```python
from build123d import *

# Parameters (mm, degrees)
SKETCH_2_W        = 3
SKETCH_2_H        = 6
EXTRUDE_660_DEPTH = 5


with BuildPart() as part:
    # Sketch 202 → Revolve 495 (revolve)
    with BuildSketch(Plane.XY, mode=Mode.PRIVATE) as revolve_495_sk:
        with BuildLine():
            Line((15, 0), (13, 0))
            Line((13, 0), (6, 10))
            Line((6, 10), (0, 10))
            Line((0, 10), (0, 286.3))
            Line((0, 286.3), (10, 286.3))
            ThreePointArc((10, 286.3), (14.127651137, 284.674598502), (18, 282.510262985))
            Line((18, 282.510262985), (18, 285.510262985))
            Line((18, 285.510262985), (20, 285.510262985))
            Line((20, 285.510262985), (20, 281.10043911))
            ThreePointArc((20, 281.10043911), (29.571946165, 269.497448129), (33, 254.851629613))
            Line((33, 254.851629613), (33, 39.851629613))
            ThreePointArc((33, 39.851629613), (27.867639585, 22.176939688), (14.066990064, 10))
            Line((14.066990064, 10), (15, 0))
        make_face()
    revolve(revolve_495_sk.sketch.rotate(Axis((0, 0, 0), (0, 1, 0)), 90), axis=Axis((0, 0, 0), (0, 1, 0)))

    # Эскиз2 → Extrude 660 (add)
    with BuildSketch(Plane(origin=(0, 285.510262985, 0), x_dir=(1, 0, 0), z_dir=(0, 1, 0))):
        with Locations((19.5, 0)):
            Rectangle(SKETCH_2_W, SKETCH_2_H)
    extrude(amount=-EXTRUDE_660_DEPTH)


solid = part.part
```
Check sheet for the modelled part. Datum: model origin and axes. Units: mm. A direction names the side the tool comes from. Round coordinates to 2 decimals unless told otherwise and drop trailing zeros. Loops run counter-clockwise (first coordinate to the right, second up) from the corner with the lowest first, then second, coordinate; pieces in that order, holes last. Notation, with made-up numbers: (-19.5, 44.5) - (4.5, 44.5) arc R26 ccw to (4.5, 60.5) - close; hole circle Ø5 at (4.5, 11.5). An arc over 180 degrees is marked (long way). Write item = value, one per line. Start each with the question number.
Q1. Depth check by flat-ended pin: P1, Ø12, axis at x = 23, z = -25.5, coming from the +Y side; P2, Ø3.5, axis at x = 1.5, z = 1, coming from the -Y side; P3, Ø4, axis at y = 135, z = 16, coming from the -X side. Enter the tip coordinate at first touch or a pass-through.
Q2. Release check for a two-part mould opening along X. For faces 5 (the face through (-19.982, 283.274, -0.837)), 6 (the face through (8, 285.51, -16.4)), 7 (the face through (6.189, 9.514, 1.374)), 8 (the face through (-12.165, 284.031, 13.267)) record: pulls with the +X half, pulls with the -X half, needs draft (parallel to the pull), parting line crosses it, or undercut.
Q3. Access from +Z, -Z, +X, -X, +Y, -Y to the whole of each face (thin tool, end or side, straight path). Record for faces 1 (the face through (21, 283, 0)), 2 (the face through (0, 10, 0)), 3 (the face through (-9.912, 145.847, -31.476)), 4 (the face through (-4.34, 6.04, -13.77)).
Q4. Thickness scan on L1, parallel to X at y = 284, z = 0; L2, parallel to X at y = 283.5, z = 0; L3, parallel to Y at x = 3, z = -12. Record the ranges inside material, lowest first.
Q5. Section check A-A (x = 0). Record the boundary of the cut face in (y, z).
Q6. Section check C-C (z = 0). Record the boundary of the cut face in (x, y).
Q7. Section check B-B (y = 221.5). Record the boundary of the cut face in (x, z), plus the area to 3 significant figures.
Q8. Section check D-D (x = -22.5). Record the boundary of the cut face in (y, z), plus the area to 3 significant figures.
Derived:
q1.P1 = 271.76
q1.P2 = 10
q1.P3 = -29.88
q2.face_5 = parting line crosses it
q2.face_6 = needs draft
q2.face_7 = undercut
q2.face_8 = undercut
q3.face_1 = +Z, -Z, +X, +Y
q3.face_2 = -Y
q3.face_3 = +Y, -Y
q3.face_4 = none
q4.L1 = -20 to -18, -15.47 to 15.47, 18 to 21
q4.L2 = -20 to -18, -16.38 to 16.38, 18 to 21
q4.L3 = 0.9 to 285.45
q5.outline = (0, -15) - (10, -14.07) arc R33 ccw to (39.85, -33) - (254.85, -33) arc R33 ccw to (281.1, -20) - (285.51, -20) - (285.51, -18) - (282.51, -18) arc R33 ccw to (286.3, -10) - (286.3, 10) arc R33 ccw to (282.51, 18) - (285.51, 18) - (285.51, 20) - (281.1, 20) arc R33 ccw to (254.85, 33) - (39.85, 33) arc R33 ccw to (10, 14.07) - (0, 15) - (0, 13) - (10, 6) - (10, -6) - (0, -13) - close
q6.outline = (-33, 39.85) arc R33 ccw to (-14.07, 10) - (-15, 0) - (-13, 0) - (-6, 10) - (6, 10) - (13, 0) - (15, 0) - (14.07, 10) arc R33 ccw to (33, 39.85) - (33, 254.85) arc R33 ccw to (20.75, 280.51) - (21, 280.51) - (21, 285.51) - (18, 285.51) - (18, 282.51) arc R33 ccw to (10, 286.3) - (-10, 286.3) arc R33 ccw to (-18, 282.51) - (-18, 285.51) - (-20, 285.51) - (-20, 281.1) arc R33 ccw to (-33, 254.85) - close
q7.outline = circle Ø66 at (0, 0)
q7.area = 3,420 mm^2
q8.outline = (39.85, -24.14) - (254.85, -24.14) arc R24.14 ccw to (254.85, 24.14) - (39.85, 24.14) arc R24.14 ccw to start
q8.area = 12,200 mm^2
